Input: dimensioned drawing with shaded views. Units: mm. Origin: part minimum x, y, z. A direction names the side the tool comes from. Give positions to 0.01 mm unless a question says otherwise; leave off trailing zeros. Loops run counter-clockwise (first coordinate to the right, second up) from the corner with the lowest first, then second, coordinate; pieces in that order, holes last.
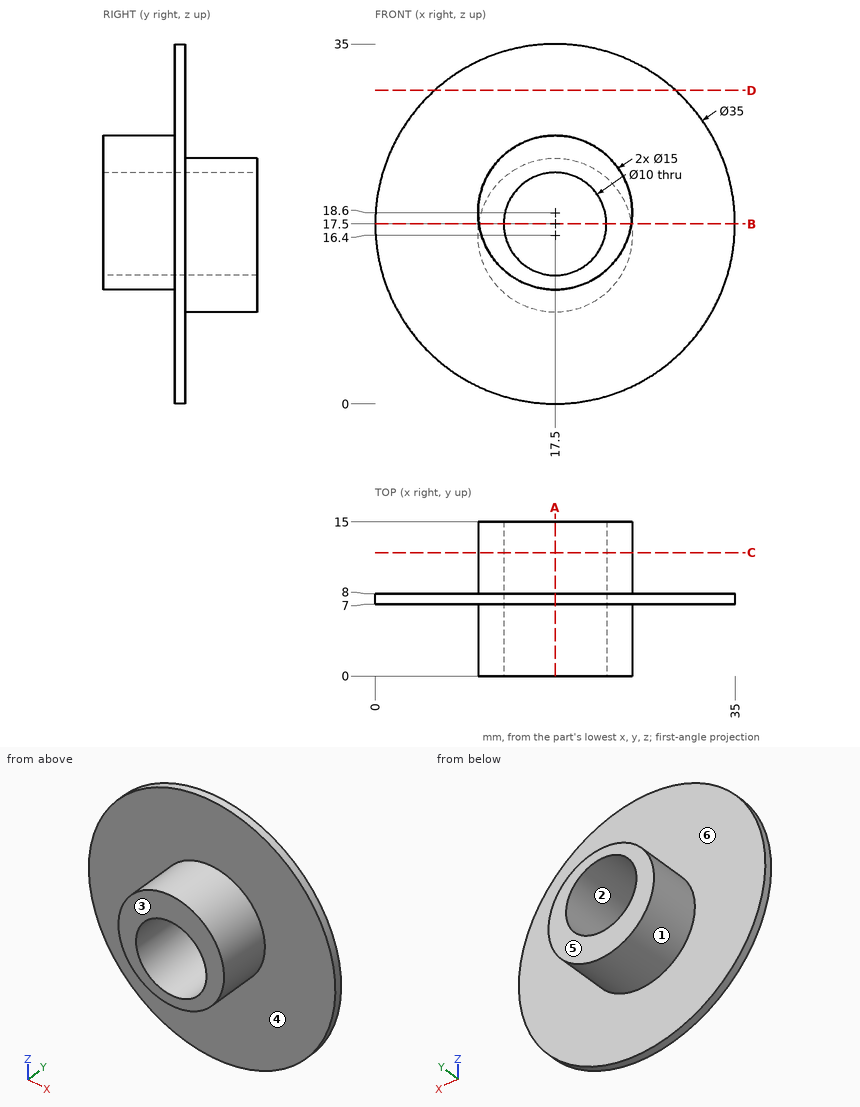
Item 1: Ray query, probe 1 along Y at (x, z) = (17, 6.5); probe 2 along X at (y, z) = (5, 18.5); probe 3 along X at (y, z) = (6, 17.5). Return the intervals inside material, ascending.
Values follow:
probe 1: y = 7 to 8
probe 2: x = 10 to 12.6, 22.4 to 25
probe 3: x = 10.08 to 12.5, 22.5 to 24.92
Item 2: Section query B-B on z = 17.5. Return loops of the section in (x, y), plus the area to 3 significant figures.
Values follow:
outline: (0, 7) - (10.08, 7) - (10.08, 0) - (12.5, 0) - (12.5, 15) - (10.08, 15) - (10.08, 8) - (0, 8) - close; (22.5, 0) - (24.92, 0) - (24.92, 7) - (35, 7) - (35, 8) - (24.92, 8) - (24.92, 15) - (22.5, 15) - close
area: 92.7 mm2
Item 3: Pin query (flat end, axial travel): pin 1 (8 mm diameter, centred on y = 8.5, z = 29.5, fed in from -X); pin 2 (1 mm diameter, centred on x = 26, y = 9.5, fed in from -Z); pin 3 (2 mm diameter, centred on x = 4.5, z = 18, fed in from -Y). Return the tip coordinate at first contact, or that it passes through.
Values follow:
pin 1: stops at x = 1.95
pin 2: passes through
pin 3: stops at y = 7
Item 4: Section query A-A on x = 17.5. Return loops of the section in (y, z), plus the area to 3 significant figures.
Values follow:
outline: (0, 11.1) - (7, 11.1) - (7, 0) - (8, 0) - (8, 8.9) - (15, 8.9) - (15, 12.5) - (0, 12.5) - close; (0, 22.5) - (15, 22.5) - (15, 23.9) - (8, 23.9) - (8, 35) - (7, 35) - (7, 26.1) - (0, 26.1) - close
area: 95.0 mm2
Item 5: Draft query along Z for the marked faces 1, 2 and 3. Return one class per face: +Z half, -Z half, draft (parallel to the pull), parting line (faces both ways), or undercut.
Values follow:
face 1: parting line
face 2: undercut
face 3: draft
Item 6: Section query D-D on z = 30.5. Return loops of the section in (x, y), plus the area to 3 significant figures.
Values follow:
outline: (5.78, 7) - (29.22, 7) - (29.22, 8) - (5.78, 8) - close
area: 23.4 mm2
Item 7: Set-up query: the marked faces 4, 5 and 6. Return all of +Z, -Z, +X, -X, +Y, -Y with unobstructed straight access to the full face (end or side cutting, diameter ignored); none if empty.
Values follow:
face 4: -Y
face 5: +Z, -Z, +X, -X, +Y
face 6: +Y
Item 8: Section query C-C on y = 12. Return loops of the section in (x, z), plus the area to 3 significant figures.
Values follow:
outline: circle Ø15 at (17.5, 16.4); hole circle Ø10 at (17.5, 17.5)
area: 98.2 mm2
